```python
from build123d import *

# Parameters (mm, degrees)
SKETCH1_R           = 1.5
SKETCH1_R_2         = 1
BOSS_EXTRUDE1_DEPTH = 3


with BuildPart() as part:
    # Sketch1 → Boss-Extrude1 (new body)
    with BuildSketch(Plane.XY):
        with BuildLine():
            Line((0, 0), (22, 0))
            Line((22, 0), (22.223388106, 0))
            ThreePointArc((22.223388106, 0), (22.930494887, -0.292893219), (23.223388106, -1))
            Line((23.223388106, -1), (23.223388106, -6.271970615))
            ThreePointArc((23.223388106, -6.271970615), (18.521001308, -13.695477275), (10.2692294, -10.674028436))
            ThreePointArc((10.2692294, -10.674028436), (7.057961936, -9.471675777), (3.827272257, -10.620821039))
            ThreePointArc((3.827272257, -10.620821039), (-5.644684501, -8.034093627), (0, 0))
        make_face()
        with Locations((0, -6)):
            Circle(SKETCH1_R, mode=Mode.SUBTRACT)
        with Locations((19.690645816, -4.936162338)):
            Circle(SKETCH1_R_2, mode=Mode.SUBTRACT)
        with Locations((16.268762771, -9.747966239)):
            Circle(SKETCH1_R, mode=Mode.SUBTRACT)
    extrude(amount=BOSS_EXTRUDE1_DEPTH)


solid = part.part
```
Geometry check sheet. Reference: the model listing, model coordinates, mm. A direction names the side the tool comes from. Coordinates: 2 decimals unless noted, no trailing zeros. Order: outer loops, then holes, each group sorted by start corner. A loop starts at its lowest first (then second) coordinate and runs counter-clockwise, first axis right, second up.
Item 1: Section check A-A (x = 19). Enter the section's corners in (y, z).
Item 2: Depth check by flat-ended pin: pin 1 (2.5 mm diameter, centred on x = 0, y = -6, fed in from +Z); pin 2 (0.9 mm diameter, centred on y = -4, z = 2, fed in from +X); pin 3 (1 mm diameter, centred on y = -9.5, z = 2, fed in from +X). Enter the tip coordinate at first touch or a pass-through.
Item 3: Section check B-B (z = 1.1). Enter the section's corners in (x, y), plus the area to 3 significant figures.
Item 4: Mould release check, pull along X, two halves, no side actions. Record for faces 1 (the cylindrical face through (22.923, -0.285, 1.479)), 2 (the cylindrical face through (7.107, -9.472, 1.479)), 3 (the flat face through (9, -5, 3)): released by +X, released by -X, zero draft, split by the parting line, or undercut.
Item 5: Section check C-C (y = -13). Enter the section's corners in (x, z).
Item 6: Section check D-D (x = -3). Enter the section's corners in (y, z).
Item 7: Scan lines: line 1 along Y through (x, z) = (16.25, 1.4); line 2 along Y through (x, z) = (7, 1.55); line 3 along X through (y, z) = (-6.5, 2.15). Record each from-to range of solid material in increasing order.
Item 8: Tool access check on faces 4 (the cylindrical face through (-5.59, -8.18, 1.48)), 5 (the flat face through (23.223, -4, 1)). Record the directions out of +Z, -Z, +X, -X, +Y, -Y that give a thin tool (end or side, any length) a straight path to the whole face; none if there is none.
Check sheet entries:
1. outline: (-13.51, 0) - (-5.66, 0) - (-5.66, 3) - (-13.51, 3) - close; (-4.21, 0) - (0, 0) - (0, 3) - (-4.21, 3) - close
2. pin 1: passes through
2. pin 2: stops at x = 23.22
2. pin 3: stops at x = 23
3. outline: (0, 0) arc R6 ccw (long way) to (3.83, -10.62) arc R5 cw to (10.27, -10.67) arc R7 ccw to (23.22, -6.27) - (23.22, -1) arc R1 ccw to (22.22, 0) - close; hole circle Ø3 at (0, -6); hole circle Ø3 at (16.27, -9.75); hole circle Ø2 at (19.69, -4.94)
3. area: 313 mm2
4. face 1: released by +X
4. face 2: undercut
4. face 3: zero draft
5. outline: (12.55, 0) - (19.98, 0) - (19.98, 3) - (12.55, 3) - close
6. outline: (-11.2, 0) - (-0.8, 0) - (-0.8, 3) - (-11.2, 3) - close
7. line 1: y = -14.07 to -11.25, -8.25 to 0
7. line 2: y = -9.47 to 0
7. line 3: x = -5.98 to -1.41, 1.41 to 23.25
8. face 4: +Z, -Z
8. face 5: +Z, -Z, +X, +Y
